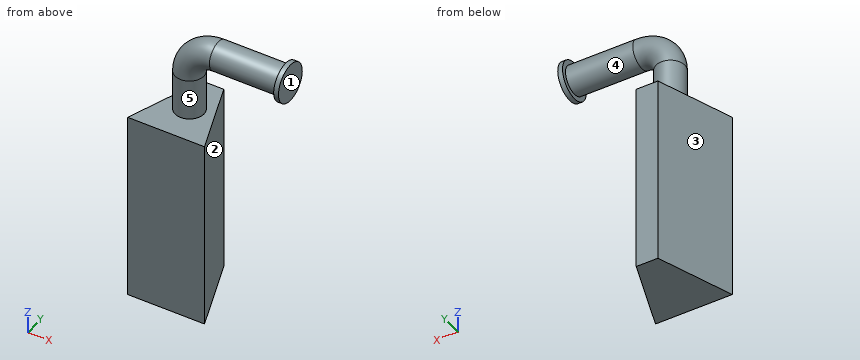
```python
from build123d import *

# Parameters (mm, degrees)
BOSS_EXTRUDE1_DEPTH = 40
SKETCH4_R           = 3
SKETCH5_R           = 4
BOSS_EXTRUDE2_DEPTH = 1


with BuildPart() as part:
    # Sketch1 → Boss-Extrude1 (new body)
    with BuildSketch(Plane.XY):
        Polygon((15.979053375, 0), (10.246522185, 15.75), (5.73253119, 15.75), (0, 0), align=None)
    extrude(amount=BOSS_EXTRUDE1_DEPTH)

    # Sweep1: sweep along a path in Sketch3
    with BuildLine(Plane(origin=(0, 7.875, 0), x_dir=(-1, 0, 0), z_dir=(0, -1, 0))) as sweep1_path:
        Line((-7.989526687, -40), (-7.989526687, -48.56216486))
        ThreePointArc((-7.989526687, -48.56216486), (-9.746886, -52.804805547), (-13.989526687, -54.56216486))
        Line((-13.989526687, -54.56216486), (-27.989526687, -54.56216486))
    # Sketch4 → Sweep1 (sweep)
    with BuildSketch(Plane(origin=(27.989526687, 0, 0), x_dir=(0, 0, -1), z_dir=(1, 0, 0))):
        with Locations((-54.56216486, 7.875)):
            Circle(SKETCH4_R)
    sweep(path=sweep1_path.line)

    # Sketch5 → Boss-Extrude2 (add)
    with BuildSketch(Plane(origin=(27.989526687, 0, 0), x_dir=(0, 0, -1), z_dir=(1, 0, 0))):
        with Locations((-54.56216486, 7.875)):
            Circle(SKETCH5_R)
    extrude(amount=BOSS_EXTRUDE2_DEPTH)


solid = part.part
```
Here's how the part is built. I have some questions about the finished solid (model axes, mm). Face numbers are marked on the shaded views. A direction names the side the tool comes from. Give positions to 0.01 mm unless a question says otherwise; leave off trailing zeros. Order: outer loops, then holes, each group sorted by start corner. A loop starts at its lowest first (then second) coordinate and runs counter-clockwise, first axis right, second up. Notation, with made-up numbers: (-21, 5) -> (9, 5) arc R31 cw to (9, 34) -> close; hole circle Ø11 at (61, 89.5). An arc over 180 degrees is marked (long way). Use CSV: the item, a comma, the result in double quotes. Start each with the question number.
Item 1: Suppose I cut it at B-B (z = 6). List the corners of the cut face in (x, y) for me.
Item 2: Suppose I cut it at D-D (x = 23.5). List the corners of the cut face in (y, z) for me (3 decimals), and give its area (3 significant figures).
Item 3: Thinking about a two-plate mould opening in X: for the marked faces 3, 4 and 5, which applies, pulls with the +X half, pulls with the -X half, needs draft (parallel to the pull), parting line crosses it, or undercut?
Item 4: Suppose I cut it at C-C (y = 14). List the corners of the cut face in (x, z) for me, and give its area (3 significant figures).
Item 5: Suppose I cut it at A-A (x = 15.25). List the corners of the cut face in (y, z) for me (3 decimals), and give its area (3 significant figures).
Item 6: If I drill on probe 1 along Z at (x, y) = (23.5, 8); probe 2 along Z at (x, y) = (6.75, 11); probe 3 along X at (y, z) = (12, 35.5), over which ranges is the centre line in solid material (lowest first)? Write a range as [from, to].
Item 7: On a 3-axis mill with a long thin cutter (end or side, diameter ignored), from which of +Z, -Z, +X, -X, +Y, -Y can I reach the whole of each face in a straight line? I mean the marked faces 1 and 2. Say none if no direction works.
Item 8: I'm going to push flat-ended pins straight in: P1, Ø4, axis at x = 4, y = 2.5, coming from the +Z side; P2, Ø9, axis at y = 8.5, z = 53, coming from the -X side; P3, Ø4, axis at x = 14.5, y = 13.5, coming from the -Z side; P4, Ø8, axis at x = 22, y = 12.5, coming from the -Z side. Where does each tip first touch, or does it pass through?
Answer block:
1,outline,"(0, 0) -> (15.98, 0) -> (10.25, 15.75) -> (5.73, 15.75) -> close"
2,outline,"circle Ø6 at (7.875, 54.562)"
2,area,"28.3 mm^2"
3,face 3,"pulls with the -X half"
3,face 4,"undercut"
3,face 5,"parting line crosses it"
4,outline,"(5.1, 0) -> (10.88, 0) -> (10.88, 40) -> (5.1, 40) -> close"
4,area,"232 mm^2"
5,outline,"(0, 0) -> (2.003, 0) -> (2.003, 40) -> (0, 40) -> close; circle Ø6 at (7.875, 54.562)"
5,area,"108 mm^2"
6,probe 1,"z = [51.56, 57.56]"
6,probe 2,"z = [0, 40]"
6,probe 3,"x = [4.37, 11.61]"
7,face 1,"+Z, -Z, +X, +Y, -Y"
7,face 2,"-Z, +X, +Y"
8,P1,"stops at z = 40"
8,P2,"stops at x = 4.99"
8,P3,"passes through"
8,P4,"stops at z = 51.63"
